from build123d import *

# Parameters (mm, degrees)
SKETCH1_W           = 59
SKETCH1_H           = 30
BOSS_EXTRUDE1_DEPTH = 30
SKETCH2_R           = 2.5
SKETCH2_R_2         = 3.5
CUT_EXTRUDE1_DEPTH  = 52.674461778


with BuildPart() as part:
    # Sketch1 → Boss-Extrude1 (new body)
    with BuildSketch(Plane.XY):
        Rectangle(SKETCH1_W, SKETCH1_H)
        Polygon((4, 2.727207794), (6.572792206, 5.3), (8, 5.3), (8, 3.1), (10, 5.1), (10, 10), (5.1, 10), (3.1, 8), (5.3, 8), (5.3, 6.572792206), (2.727207794, 4), (-2.727207794, 4), (-5.3, 6.572792206), (-5.3, 8), (-3.1, 8), (-5.1, 10), (-10, 10), (-10, 5.1), (-8, 3.1), (-8, 5.3), (-6.572792206, 5.3), (-4, 2.727207794), (-4, -2.727207794), (-6.572792206, -5.3), (-8, -5.3), (-8, -3.1), (-10, -5.1), (-10, -10), (-5.1, -10), (-3.1, -8), (-5.3, -8), (-5.3, -6.572792206), (-2.727207794, -4), (2.727207794, -4), (5.3, -6.572792206), (5.3, -8), (3.1, -8), (5.1, -10), (10, -10), (10, -5.1), (8, -3.1), (8, -5.3), (6.572792206, -5.3), (4, -2.727207794), align=None, mode=Mode.SUBTRACT)
    extrude(amount=-BOSS_EXTRUDE1_DEPTH)

    # Sketch2 → Cut-Extrude1 (cut, through all)
    with BuildSketch(Plane(origin=(0, 15, 0), x_dir=(1, 0, 0), z_dir=(0, 1, 0))):
        with Locations(Location((0, 10, 0), (0, 0, 270))):
            Circle(SKETCH2_R)
        with Locations(Location((0, 20, 0), (0, 0, 270))):
            Circle(SKETCH2_R)
        with Locations(Location((-23, 24.5, 0), (0, 0, 270))):
            Circle(SKETCH2_R_2)
        with Locations(Location((23, 24.5, 0), (0, 0, 270))):
            Circle(SKETCH2_R_2)
        with Locations(Location((22.450748844, 11.5, 0), (0, 0, 270))):
            Circle(SKETCH2_R_2)
        with Locations(Location((-23, 11.5, 0), (0, 0, 270))):
            Circle(SKETCH2_R_2)
    extrude(amount=-CUT_EXTRUDE1_DEPTH, mode=Mode.SUBTRACT)


solid = part.part
Build history of the part. All positions in model axes, mm. Give positions to 0.01 mm unless a question says otherwise; leave off trailing zeros. Loops run counter-clockwise (first coordinate to the right, second up) from the corner with the lowest first, then second, coordinate; pieces in that order, holes last. Notation, with made-up numbers: (50.5, 12.25) - (96.5, 12.25) arc R30 ccw to (96.5, 34.25) - close; hole circle Ø8 at (-15, -38.75). An arc over 180 degrees is marked (long way). Write item = value, one per line. Start each with the question number.
1) Band-saw the part on A-A on x = -23. Give the cut face in (y, z).
2) Band-saw the part on B-B on x = 0. Give the cut face in (y, z), plus the area to 3 significant figures.
3) Band-saw the part on C-C on y = 12. Give the cut face in (x, z).
4) Pull direction Z, two halves, no side cores. Call faces 1 (the cylindrical face through (-20.05, 0.21, -22.62)), 2 (the flat face through (0, 7, 0)), 3 (the flat face through (0, -4, -15)): +Z half, -Z half, draft (parallel to the pull), parting line (faces both ways), or undercut.
5) Band-saw the part on D-D on z = -10.25. Count the separate pieces of the cut face and the enclosed holes in it, plus the area to 3 significant figures.
6) Probe probe 1 along X at (y, z) = (0.5, -24.5); probe 2 along Y at (x, z) = (-7.5, -15); probe 3 along X at (y, z) = (12.75, -20). List the from-to ranges inside material, lowest first. Write a range as from..to.
7) Drop a flat-ended pin along its axis: pin 1 Ø3 at (x, y) = (-14, -3) entering from +Z. Give the stop position or say it passes through.
Final values:
q1.outline = (-15, -30) - (15, -30) - (15, -28) - (-15, -28) - close; (-15, -21) - (15, -21) - (15, -15) - (-15, -15) - close; (-15, -8) - (15, -8) - (15, 0) - (-15, 0) - close
q2.outline = (-15, -30) - (-4, -30) - (-4, -22.5) - (-15, -22.5) - close; (-15, -17.5) - (-4, -17.5) - (-4, -12.5) - (-15, -12.5) - close; (-15, -7.5) - (-4, -7.5) - (-4, 0) - (-15, 0) - close; (4, -30) - (15, -30) - (15, -22.5) - (4, -22.5) - close; (4, -17.5) - (15, -17.5) - (15, -12.5) - (4, -12.5) - close; (4, -7.5) - (15, -7.5) - (15, 0) - (4, 0) - close
q2.area = 440 mm²
q3.outline = (-29.5, -30) - (29.5, -30) - (29.5, 0) - (-29.5, 0) - close; hole circle Ø7 at (-23, -24.5); hole circle Ø7 at (-23, -11.5); hole circle Ø5 at (0, -20); hole circle Ø5 at (0, -10); hole circle Ø7 at (22.45, -11.5); hole circle Ø7 at (23, -24.5)
q4.face_1 = undercut
q4.face_2 = +Z half
q4.face_3 = draft
q5.separate_pieces = 4
q5.enclosed_holes = 0
q5.area = 1,080 mm²
q6.probe_1 = -29.5..-26.5, -19.5..-4, 4..19.5, 26.5..29.5
q6.probe_2 = -15..-10, -5.3..5.3, 10..15
q6.probe_3 = -29.5..-2.5, 2.5..29.5
q7.pin_1 = 0
